from build123d import *

# Parameters (mm, degrees)
F0_W     = 2.344617017
F0_H     = 7.7176926169
F0_H_2   = 0.5861528073
F1_DEPTH = 10


with BuildPart() as f1:
    # F0 (on Front) → F1 (new body)
    with BuildSketch(Plane.XZ):
        Polygon((0, 4.7380755195), (1.1234623608, 4.7380755195), (1.1234623608, 19.4407690205), (-0.1221147261, 21.2480772879), (-1.367691813, 19.4407690205), (-1.367691813, 4.7380755195), align=None)
        Polygon((1.1723085085, 4.1519227121), (1.1723085085, 3.5657699048), (4.4450012058, 3.5657699048), (4.4450012058, 4.7380755195), (1.1234623608, 4.7380755195), (0, 4.7380755195), (-1.367691813, 4.7380755195), (-4.4450012058, 4.7380755195), (-4.4450012058, 3.5657699048), (-1.1723085085, 3.5657699048), (-1.1723085085, 4.1519227121), align=None)
        with Locations((0, -0.2930764037)):
            Rectangle(F0_W, F0_H)
        with Locations((0, 3.8588463084)):
            Rectangle(F0_W, F0_H_2)
    extrude(amount=F1_DEPTH)


solid = f1.part
Part model, mm, in its own coordinate system. A direction names the side the tool comes from. Coordinates: 2 decimals unless noted, no trailing zeros. Write each loop counter-clockwise with the first axis right and the second up, starting at its lowest first coordinate (ties: lowest second). Pieces come first, ordered by that corner, then holes. Notation, with made-up numbers: (60.5, 1) - (70.5, 1) arc R18 cw to (70.5, 22) - close; hole circle Ø11 at (28.5, 8). An arc over 180 degrees is marked (long way). Put each result on its own line as item: value.
1. Probe line 1 along Z through (x, y) = (1.25, -7.5); line 2 along X through (y, z) = (-3.25, 10.75); line 3 along X through (y, z) = (-1, -1). List the from-to ranges inside material, lowest first. Write a range as [from, to].
Final values:
line 1: z = [3.57, 4.74]
line 2: x = [-1.37, 1.12]
line 3: x = [-1.17, 1.17]
2. Band-saw the part on B-B (z = 5.75). Write the cut outline in (x, y), then the cut area to 3 significant figures.
Final values:
outline: (-1.37, -10) - (1.12, -10) - (1.12, 0) - (-1.37, 0) - close
area: 24.9 mm²
3. Flat gauge pins, fed straight in: pin 1 Ø3.5 at (x, y) = (-2.5, -2.5) entering from +Z; pin 2 Ø1.5 at (x, y) = (2.5, -7) entering from -Z; pin 3 Ø1 at (x, y) = (3.5, -4) entering from +Z. Where does each tip first touch, or does it go through?
Final values:
pin 1: stops at z = 20.34
pin 2: stops at z = 3.57
pin 3: stops at z = 4.74
4. Band-saw the part on A-A (y = -7.5). Write the cut outline in (x, z) (3 decimals), then the cut area to 3 significant figures.
Final values:
outline: (-4.445, 3.566) - (-1.172, 3.566) - (-1.172, -4.152) - (1.172, -4.152) - (1.172, 3.566) - (4.445, 3.566) - (4.445, 4.738) - (1.123, 4.738) - (1.123, 19.441) - (-0.122, 21.248) - (-1.368, 19.441) - (-1.368, 4.738) - (-4.445, 4.738) - close
area: 67.4 mm²
5. 3-axis set-ups, long thin cutter, end or side, ignore diameter. For faces 1 (the flat face through (-1.368, -5, 12)), 2 (the flat face through (1.172, -5, 0)), 3 (the flat face through (-1.172, -5, 0)), 4 (the flat face through (0, 0, 8)), 5 (the flat face through (1.123, -5, 12)): which of +Z, -Z, +X, -X, +Y, -Y reach the whole face in a straight line?
Final values:
face 1: +Z, -X, +Y, -Y
face 2: -Z, +X, +Y, -Y
face 3: -Z, -X, +Y, -Y
face 4: +Z, -Z, +X, -X, +Y
face 5: +Z, +X, +Y, -Y
6. Band-saw the part on C-C (x = 2.75). Write the cut outline in (y, z), then the cut area to 3 significant figures.
Final values:
outline: (-10, 3.57) - (0, 3.57) - (0, 4.74) - (-10, 4.74) - close
area: 11.7 mm²
